from build123d import *

# Parameters (mm, degrees)
SKETCH1_R            = 1.5
BOSS_EXTRUDE1_DEPTH  = 1.55
SKETCH3_W            = 14
SKETCH3_H            = 14
BOSS_EXTRUDE2_DEPTH  = 1.55
CUT_EXTRUDE1_REACH   = 63.684
BOSS_EXTRUDE3_DEPTH  = 3.15
SKETCH3_4_W          = 5
SKETCH3_4_H          = 25
BOSS_EXTRUDE4_DEPTH  = 2
SKETCH3_5_W          = 5
SKETCH3_5_H          = 10.5
BOSS_EXTRUDE5_DEPTH  = 8.9
SKETCH3_6_W          = 6.6
SKETCH3_6_H          = 6
BOSS_EXTRUDE6_DEPTH  = 2.25
SKETCH3_7_W          = 10
SKETCH3_7_H          = 4.3
BOSS_EXTRUDE7_DEPTH  = 1.55
SKETCH5_W            = 81.6
SKETCH5_H            = 54.57
BOSS_EXTRUDE8_DEPTH  = 3.6
SKETCH5_3_W          = 1.5
SKETCH5_3_H          = 54.57
BOSS_EXTRUDE9_DEPTH  = 3.4
SKETCH6_W            = 84.6
SKETCH6_H            = 54.57
BOSS_EXTRUDE10_DEPTH = 0.8
SKETCH5_4_W          = 6
SKETCH5_4_H          = 6
BOSS_EXTRUDE11_DEPTH = 4
SKETCH5_5_W          = 12.1
SKETCH5_5_H          = 12
BOSS_EXTRUDE12_DEPTH = 6.4
SKETCH5_6_R          = 4.575
BOSS_EXTRUDE13_DEPTH = 4.55
SKETCH7_R            = 1
CUT_EXTRUDE2_DEPTH   = 3
SKETCH8_R            = 3.425
BOSS_EXTRUDE14_DEPTH = 5.45
SKETCH10_R           = 1.575
SKETCH9_R            = 1.725
FILLET1_R            = 0.2
SKETCH11_W           = 2.8
SKETCH11_H           = 23.97
CUT_EXTRUDE3_DEPTH   = 12.5
FILLET2_R            = 1
SKETCH13_W           = 84.6
SKETCH13_H           = 0.2
SKETCH13_W_2         = 81.6
CUT_EXTRUDE4_DEPTH   = 0.2
SKETCH14_W           = 81.6
SKETCH14_H           = 0.2
CUT_EXTRUDE5_DEPTH   = 0.2
SKETCH15_R           = 2.75
CUT_EXTRUDE6_DEPTH   = 1


with BuildPart() as part:
    # Sketch1 → Boss-Extrude1 (new body)
    with BuildSketch(Plane.XY):
        with BuildLine():
            Line((-53, 27.885), (53, 27.885))
            ThreePointArc((53, 27.885), (54.414213562, 27.299213562), (55, 25.885))
            Line((55, 25.885), (55, -25.885))
            ThreePointArc((55, -25.885), (54.414213562, -27.299213562), (53, -27.885))
            Line((53, -27.885), (-53, -27.885))
            ThreePointArc((-53, -27.885), (-54.414213562, -27.299213562), (-55, -25.885))
            Line((-55, -25.885), (-55, 25.885))
            ThreePointArc((-55, 25.885), (-54.414213562, 27.299213562), (-53, 27.885))
        make_face()
        with Locations(Location((-51.88, 24.715, 0), (0, 0, 180))):
            Circle(SKETCH1_R, mode=Mode.SUBTRACT)
        with Locations(Location((51.88, 24.715, 0), (0, 0, 180))):
            Circle(SKETCH1_R, mode=Mode.SUBTRACT)
        with Locations(Location((51.88, -24.715, 0), (0, 0, 180))):
            Circle(SKETCH1_R, mode=Mode.SUBTRACT)
        with Locations(Location((-51.88, -24.715, 0), (0, 0, 180))):
            Circle(SKETCH1_R, mode=Mode.SUBTRACT)
    extrude(amount=BOSS_EXTRUDE1_DEPTH)

    # Sketch3 → Boss-Extrude2 (add)
    with BuildSketch(Plane(origin=(0, 0, 0), x_dir=(-1, 0, 0), z_dir=(0, 0, -1))):
        with Locations((22, 3.885)):
            Rectangle(SKETCH3_W, SKETCH3_H)
    extrude(amount=BOSS_EXTRUDE2_DEPTH)

    # Sketch4 → Cut-Extrude1 (cut, up to next)
    with BuildSketch(Plane(origin=(0, 0, 0), x_dir=(-1, 0, 0), z_dir=(0, 0, -1)), mode=Mode.PRIVATE) as cut_extrude1_sk1:
        with BuildLine():
            Line((-10.6, 9.735), (-10.6, -9.965))
            ThreePointArc((-10.6, -9.965), (-11.75, -11.115), (-12.9, -9.965))
            Line((-12.9, -9.965), (-12.9, 9.735))
            ThreePointArc((-12.9, 9.735), (-11.75, 10.885), (-10.6, 9.735))
        make_face()
    cut_extrude1_tool1 = extrude(cut_extrude1_sk1.sketch, amount=-CUT_EXTRUDE1_REACH, mode=Mode.PRIVATE) & part.part
    add(cut_extrude1_tool1.solids().sort_by_distance((11.75, -0.115, 0))[0], mode=Mode.SUBTRACT)

    # Sketch3<3> → Boss-Extrude3 (add)
    with BuildSketch(Plane(origin=(0, 0, 0), x_dir=(-1, 0, 0), z_dir=(0, 0, -1))):
        Polygon((43.7, 11.665), (46.3, 14.265), (54.6, 14.265), (54.6, -12.685), (38, -12.685), (38, 11.665), align=None)
    extrude(amount=BOSS_EXTRUDE3_DEPTH)

    # Sketch3<4> → Boss-Extrude4 (add)
    with BuildSketch(Plane(origin=(0, 0, 0), x_dir=(-1, 0, 0), z_dir=(0, 0, -1))):
        with Locations((4.1, 0.415)):
            Rectangle(SKETCH3_4_W, SKETCH3_4_H)
    extrude(amount=BOSS_EXTRUDE4_DEPTH)

    # Sketch3<5> → Boss-Extrude5 (add)
    with BuildSketch(Plane(origin=(0, 0, 0), x_dir=(-1, 0, 0), z_dir=(0, 0, -1))):
        with Locations((-32.4, 1.335)):
            Rectangle(SKETCH3_5_W, SKETCH3_5_H)
    extrude(amount=BOSS_EXTRUDE5_DEPTH)

    # Sketch3<6> → Boss-Extrude6 (add)
    with BuildSketch(Plane(origin=(0, 0, 0), x_dir=(-1, 0, 0), z_dir=(0, 0, -1))):
        with Locations((-18.55, 1.885)):
            Rectangle(SKETCH3_6_W, SKETCH3_6_H)
    extrude(amount=BOSS_EXTRUDE6_DEPTH)

    # Sketch3<7> → Boss-Extrude7 (add)
    with BuildSketch(Plane(origin=(0, 0, 0), x_dir=(-1, 0, 0), z_dir=(0, 0, -1))):
        with Locations((42.8, -23.035)):
            Rectangle(SKETCH3_7_W, SKETCH3_7_H)
    extrude(amount=BOSS_EXTRUDE7_DEPTH)

    # Sketch5 → Boss-Extrude8 (add)
    # profile 1 of 2: a face of its own
    with BuildSketch(Plane.XY.offset(1.55)):
        with Locations((-5.45, 0.6)):
            Rectangle(SKETCH5_W, SKETCH5_H)
        with BuildLine():
            Line((10.6, -9.965), (10.6, 9.735))
            ThreePointArc((10.6, 9.735), (11.75, 10.885), (12.9, 9.735))
            Line((12.9, 9.735), (12.9, -9.965))
            ThreePointArc((12.9, -9.965), (11.75, -11.115), (10.6, -9.965))
        make_face(mode=Mode.SUBTRACT)
    # profile 2 of 2: a face of its own
    with BuildSketch(Plane.XY.offset(1.55)):
        with BuildLine():
            ThreePointArc((10.6, 9.735), (11.75, 10.885), (12.9, 9.735))
            Line((12.9, 9.735), (12.9, -9.965))
            ThreePointArc((12.9, -9.965), (11.75, -11.115), (10.6, -9.965))
            Line((10.6, -9.965), (10.6, 9.735))
        make_face()
    extrude(amount=BOSS_EXTRUDE8_DEPTH)

    # Sketch5<3> → Boss-Extrude9 (add)
    with BuildSketch(Plane.XY.offset(1.55)):
        with Locations((-47, 0.6)):
            Rectangle(SKETCH5_3_W, SKETCH5_3_H)
        with Locations((36.1, 0.6)):
            Rectangle(SKETCH5_3_W, SKETCH5_3_H)
    extrude(amount=BOSS_EXTRUDE9_DEPTH)

    # Sketch6 → Boss-Extrude10 (add)
    with BuildSketch(Plane.XY.offset(5.15)):
        with Locations((-5.45, 0.6)):
            Rectangle(SKETCH6_W, SKETCH6_H)
    extrude(amount=BOSS_EXTRUDE10_DEPTH)

    # Sketch5<4> → Boss-Extrude11 (add)
    with BuildSketch(Plane.XY.offset(1.55)):
        with Locations((45.2, -20.685)):
            Rectangle(SKETCH5_4_W, SKETCH5_4_H)
    extrude(amount=BOSS_EXTRUDE11_DEPTH)

    # Sketch5<5> → Boss-Extrude12 (add)
    with BuildSketch(Plane.XY.offset(1.55)):
        with Locations((45.75, -1.135)):
            Rectangle(SKETCH5_5_W, SKETCH5_5_H)
    extrude(amount=BOSS_EXTRUDE12_DEPTH)

    # Sketch5<6> → Boss-Extrude13 (add)
    with BuildSketch(Plane.XY.offset(1.55)):
        with Locations((46.525, 15.01)):
            Circle(SKETCH5_6_R)
    extrude(amount=BOSS_EXTRUDE13_DEPTH)

    # Sketch7 → Cut-Extrude2 (cut)
    with BuildSketch(Plane.XY.offset(6.1)):
        with Locations((46.525, 15.01)):
            Circle(SKETCH7_R)
    extrude(amount=-CUT_EXTRUDE2_DEPTH, mode=Mode.SUBTRACT)

    # Sketch8 → Boss-Extrude14 (add)
    with BuildSketch(Plane.XY.offset(7.95)):
        with Locations((45.75, -1.135)):
            Circle(SKETCH8_R)
    extrude(amount=BOSS_EXTRUDE14_DEPTH)

    # Sketch10 → Loft1 section 0
    with BuildSketch(Plane.XY.offset(11.85)):
        with Locations((45.2, -20.685)):
            Circle(SKETCH10_R)
    # Sketch9 → Loft1 section 1
    with BuildSketch(Plane.XY.offset(5.55)):
        with Locations((45.2, -20.685)):
            Circle(SKETCH9_R)
    loft()

    # Fillet1
    fillet1_edges = [part.edges().sort_by_distance(p)[0] for p in [
        (43.625, -20.685, 11.85),
    ]]
    fillet(fillet1_edges, radius=FILLET1_R)

    # Sketch11 → Cut-Extrude3 (cut)
    with BuildSketch(Plane.ZY.offset(54.6)):
        with Locations((-1.45, 1.1)):
            Rectangle(SKETCH11_W, SKETCH11_H)
    extrude(amount=-CUT_EXTRUDE3_DEPTH, mode=Mode.SUBTRACT)

    # Fillet2
    fillet2_edges = [part.edges().sort_by_distance(p)[0] for p in [
        (51.8, -7.135, 4.75),
        (51.8, 4.865, 4.75),
        (39.7, 4.865, 4.75),
        (39.7, -7.135, 4.75),
    ]]
    fillet(fillet2_edges, radius=FILLET2_R)

    # Sketch13 → Cut-Extrude4 (cut)
    with BuildSketch(Plane(origin=(0, 27.885, 0), x_dir=(1, 0, 0), z_dir=(0, 1, 0))):
        with Locations((-5.45, -1.65)):
            Rectangle(SKETCH13_W, SKETCH13_H)
        with Locations((-5.45, -5.05)):
            Rectangle(SKETCH13_W_2, SKETCH13_H)
    extrude(amount=-CUT_EXTRUDE4_DEPTH, mode=Mode.SUBTRACT)

    # Sketch14 → Cut-Extrude5 (cut)
    with BuildSketch(Plane.XZ.offset(26.685)):
        with Locations((-5.45, 5.05)):
            Rectangle(SKETCH14_W, SKETCH14_H)
    extrude(amount=-CUT_EXTRUDE5_DEPTH, mode=Mode.SUBTRACT)

    # Sketch15 → Cut-Extrude6 (cut)
    with BuildSketch(Plane.XY.offset(13.4)):
        with Locations((45.75, -1.135)):
            Circle(SKETCH15_R)
    extrude(amount=-CUT_EXTRUDE6_DEPTH, mode=Mode.SUBTRACT)


solid = part.part
Source: CAD feature listing. Evaluate the final solid. Frame: model axes, mm. A direction names the side the tool comes from. Give positions to 0.01 mm unless a question says otherwise; leave off trailing zeros. Write each loop counter-clockwise with the first axis right and the second up, starting at its lowest first coordinate (ties: lowest second). Pieces come first, ordered by that corner, then holes. Notation, with made-up numbers: M 19.25,-14.75 L 24.25,-14.75 A16 cw 24.25,1.25 Z; hole C 59,82.25 d2. An arc over 180 degrees is marked long. Return JSON: item names as keys, results as strings. Group by question number.
1) Draft query along X for faces 1 (the face through (45, -17.685, 4)), 2 (the face through (-42.1, 1, -1)), 3 (the face through (45.731, 14.402, 4.621)). Return one class per face: released by +X, released by -X, zero draft, split by the parting line, or undercut.
2) Cut plane A-A, the plane x = -51.88. Output: boundary loops of the cut face in (y, z) (3 decimals), then the cut area to 3 significant figures.
3) Set-up query: faces 4 (the face through (46, -7.135, 5)), 5 (the face through (42.33, -0.98, 10.64)), 6 (the face through (-46, 1, -3.15)), 7 (the face through (-46, -12.685, -2)), 8 (the face through (-6, -26.685, 3)). Return all of +Z, -Z, +X, -X, +Y, -Y with unobstructed straight access to the full face (end or side cutting, diameter ignored); none if empty.
4) Cut plane D-D, the plane z = -4.5. Output: boundary loops of the cut face in (x, y) (3 decimals).
5) First-contact query: pin 1 Ø2.5 at (y, z) = (7, -1.5) entering from -X; pin 2 Ø1.9 at (y, z) = (-0.5, 4) entering from -X; pin 3 Ø6 at (x, z) = (20.5, 8) entering from +Y (3 decimals); pin 4 Ø16.5 at (x, y) = (-5, -6.5) entering from -Z. Flat tips, straight axial feed; report the tip coordinate or a pass-through.
6) Ray query, L1, parallel to Y at x = -51.88, z = 0.35 (3 decimals); L2, parallel to X at y = 9.5, z = -1.5; L3, parallel to X at y = 1, z = 4.5. Return the intervals inside material, ascending.
7) Cut plane C-C, the plane x = 7.5. Output: boundary loops of the cut face in (y, z) (3 decimals), then the cut area to 3 significant figures.
Data:
{
 "1": {"face 1": "zero draft", "face 2": "released by -X", "face 3": "undercut"},
 "2": {"outline": "M -27.885,0 L -26.215,0 L -26.215,1.55 L -27.885,1.55 Z; M -23.215,0 L -12.685,0 L -12.685,-3.15 L 14.265,-3.15 L 14.265,0 L 23.215,0 L 23.215,1.55 L -23.215,1.55 Z; M 26.215,0 L 27.885,0 L 27.885,1.55 L 26.215,1.55 Z; hole M -10.885,-2.85 L 13.085,-2.85 L 13.085,-0.05 L -10.885,-0.05 Z", "area": "94.9 mm²"},
 "3": {"face 4": "+Z, +X", "face 5": "+Z", "face 6": "-Z, -X, +Y, -Y", "face 7": "-Z, +X, -X", "face 8": "+Z, +X, -X, -Y"},
 "4": {"outline": "M 29.9,-3.915 L 34.9,-3.915 L 34.9,6.585 L 29.9,6.585 Z"},
 "5": {"pin 1": "stops at x = -42.1", "pin 2": "stops at x = -47.75", "pin 3": "stops at y = 27.885", "pin 4": "stops at z = -2"},
 "6": {"L1": "y = -27.885 to -26.215, -23.215 to 23.215, 26.215 to 27.885", "L2": "x = -42.1 to -38, -29 to -15, -6.6 to -1.6", "L3": "x = -47.75 to 36.85, 39.7 to 51.8"},
 "7": {"outline": "M -27.885,0 L 27.885,0 L 27.885,1.55 L 27.685,1.55 L 27.685,1.75 L 27.885,1.75 L 27.885,4.95 L 27.685,4.95 L 27.685,5.15 L 27.885,5.15 L 27.885,5.95 L -26.685,5.95 L -26.685,5.15 L -26.485,5.15 L -26.485,4.95 L -26.685,4.95 L -26.685,1.55 L -27.885,1.55 Z", "area": "326 mm²"}
}
